from build123d import *

# Parameters (mm, degrees)
F0_R          = 5.08
F1_DEPTH      = 12.7
F2_R          = 2.54
F3_DEPTH      = 12.7
F4_W          = 6.35
F4_H          = 5.08
F5_DEPTH      = 12.7
F7_DEPTH      = 5.081
F7_DEPTH_BACK = 5.081
F8_R          = 1.190625
F9_DEPTH      = 5.0810001
F9_DEPTH_BACK = 5.0810001
F11_DEPTH     = 12.7
F13_DEPTH     = 12.7


with BuildPart() as f1:
    # F0 (on Top) → F1 (new body)
    with BuildSketch(Plane.XY):
        Circle(F0_R)
    extrude(amount=F1_DEPTH)

    # F2 (on face) → F3 (join)
    with BuildSketch(Plane(origin=(0, 0, 0), x_dir=(1, 0, 0), z_dir=(0, 0, -1))):
        Circle(F2_R)
    extrude(amount=F3_DEPTH)

    # F4 (on Front) → F5 (cut, symmetric)
    with BuildSketch(Plane.XZ):
        with Locations((0, 10.16)):
            Rectangle(F4_W, F4_H)
    extrude(amount=F5_DEPTH, both=True, mode=Mode.SUBTRACT)

    # F6 (on Right) → F7 (cut, two sides)
    with BuildSketch(Plane.YZ) as f7_sk:
        with BuildLine():
            ThreePointArc((1.397, 5.08), (0, 6.477), (-1.397, 5.08))
            Line((-1.397, 5.08), (-1.397, 2.54))
            ThreePointArc((-1.397, 2.54), (0, 1.143), (1.397, 2.54))
            Line((1.397, 2.54), (1.397, 5.08))
        make_face()
    extrude(amount=F7_DEPTH, mode=Mode.SUBTRACT)
    extrude(f7_sk.sketch, amount=-F7_DEPTH_BACK, mode=Mode.SUBTRACT)

    # F8 (on Right) → F9 (cut, two sides)
    with BuildSketch(Plane.YZ) as f9_sk:
        with Locations((0, 10.795)):
            Circle(F8_R)
    extrude(amount=-F9_DEPTH, mode=Mode.SUBTRACT)
    extrude(f9_sk.sketch, amount=F9_DEPTH_BACK, mode=Mode.SUBTRACT)

    # F10 (on face) → F11 (cut, symmetric)
    with BuildSketch(Plane(origin=(3.175, 0, 0), x_dir=(0, -1, 0), z_dir=(-1, 0, 0))):
        Polygon((3.965573729, 10.16), (3.965573729, 12.7), (1.905, 12.7), align=None)
        Polygon((-3.965573729, 10.16), (-1.905, 12.7), (-3.965573729, 12.7), align=None)
    extrude(amount=F11_DEPTH, both=True, mode=Mode.SUBTRACT)

    # F12 (on Front) → F13 (cut, symmetric)
    with BuildSketch(Plane.XZ):
        with BuildLine():
            Line((3.175, 7.366), (3.175, 7.62))
            Line((3.175, 7.62), (-3.175, 7.62))
            Line((-3.175, 7.62), (-3.175, 7.366))
            ThreePointArc((-3.175, 7.366), (0, 6.515261314), (3.175, 7.366))
        make_face()
    extrude(amount=F13_DEPTH, both=True, mode=Mode.SUBTRACT)


solid = f1.part
Model file for the job. Use its own axes, mm. A direction names the side the tool comes from. Give positions to 0.01 mm unless a question says otherwise; leave off trailing zeros. Loops run counter-clockwise (first coordinate to the right, second up) from the corner with the lowest first, then second, coordinate; pieces in that order, holes last. Notation, with made-up numbers: (-37.5, -12) - (-6.5, -12) arc R15 ccw to (-6.5, 15) - close; hole circle Ø10 at (-12, 45). An arc over 180 degrees is marked (long way). Use one line per item in the form item = value.
(1) Pull direction Z, two halves, no side cores. Call faces 6 (the face through (2, -2, 0)), 7 (the face through (-0.07, 0.92, 6.13)), 8 (the face through (-0.047, 1.058, 6.515)): pulls with the +Z half, pulls with the -Z half, needs draft (parallel to the pull), parting line crosses it, or undercut.
Determined:
face_6 = pulls with the -Z half
face_7 = undercut
face_8 = pulls with the +Z half
(2) Cut at C-C (z = 3). Give the cut face in (x, y), then the cut area to 3 significant figures.
Determined:
outline = (-4.88, -1.4) arc R5.08 ccw to (4.88, -1.4) - close; (-4.88, 1.4) - (4.88, 1.4) arc R5.08 ccw to start
area = 53.0 mm^2
(3) Drop flat-ended pins along their axis: P1, Ø2, axis at x = -1, y = -1, coming from the +Z side; P2, Ø1, axis at x = -1, y = 1, coming from the +Z side; P3, Ø1.6, axis at y = -1.5, z = 11.5, coming from the -X side; P4, Ø1.4, axis at y = 0, z = 10.795, coming from the -X side. Give the stop position or say it passes through.
Determined:
P1 = 6.84
P2 = 6.69
P3 = -5.03
P4 = through
(4) Drill centre lines: L1, parallel to Z at x = 4.3, y = 0; L2, parallel to Z at x = 4, y = -0.75; L3, parallel to Z at x = 0.25, y = -3.25. Where is each one in solid material? Low to high.
Determined:
L1 = 0 to 1.14, 6.48 to 9.6, 11.99 to 12.7
L2 = 0 to 1.36, 6.26 to 9.87, 11.72 to 12.7
L3 = 0 to 6.52
(5) Cut at A-A (y = 0). Give the cut face in (x, z) (3 decimals).
Determined:
outline = (-5.08, 0) - (-2.54, 0) - (-2.54, -12.7) - (2.54, -12.7) - (2.54, 0) - (5.08, 0) - (5.08, 1.143) - (-5.08, 1.143) - close; (-5.08, 6.477) - (5.08, 6.477) - (5.08, 9.604) - (3.175, 9.604) - (3.175, 7.366) arc R6.35 cw to (-3.175, 7.366) - (-3.175, 9.604) - (-5.08, 9.604) - close; (-5.08, 11.986) - (-3.175, 11.986) - (-3.175, 12.7) - (-5.08, 12.7) - close; (3.175, 11.986) - (5.08, 11.986) - (5.08, 12.7) - (3.175, 12.7) - close
(6) Cut at D-D (x = 4). Give the cut face in (y, z) (3 decimals).
Determined:
outline = (-3.132, 0) - (3.132, 0) - (3.132, 11.188) - (1.905, 12.7) - (-1.905, 12.7) - (-3.132, 11.188) - close; hole (-1.397, 2.54) arc R1.397 ccw to (1.397, 2.54) - (1.397, 5.08) arc R1.397 ccw to (-1.397, 5.08) - close; hole circle Ø2.381 at (0, 10.795)
(7) 3-axis set-ups, long thin cutter, end or side, ignore diameter. For faces 1 (the face through (0, 0, -12.7)), 2 (the face through (3.761, 2.721, 11.694)), 3 (the face through (0, -1.397, 4)), 4 (the face through (-0.33, -2.52, -6.26)), 5 (the face through (3.175, 0, 9)): which of +Z, -Z, +X, -X, +Y, -Y reach the whole face in a straight line?
Determined:
face_1 = -Z, +X, -X, +Y, -Y
face_2 = +Z, +X, -X, +Y
face_3 = +X, -X
face_4 = -Z
face_5 = +Z, +Y, -Y
(8) Cut at B-B (x = 0). Give the cut face in (y, z), then the cut area to 3 significant figures.
Determined:
outline = (-5.08, 0) - (-2.54, 0) - (-2.54, -12.7) - (2.54, -12.7) - (2.54, 0) - (5.08, 0) - (5.08, 6.52) - (-5.08, 6.52) - close; hole (-1.4, 2.54) arc R1.4 ccw to (1.4, 2.54) - (1.4, 5.08) arc R1.4 ccw to (-1.4, 5.08) - close
area = 117 mm^2
